from build123d import *

# Parameters (mm, degrees)
F1_DEPTH = 18.288
F2_W     = 17.783007
F2_H     = 7.712702
F3_DEPTH = 8.6106
F4_R     = 5.08


with BuildPart() as f1:
    # F0 (on Front) → F1 (new body)
    with BuildSketch(Plane.XZ):
        Polygon((-13.85931, 24.089288), (-28.41359, 12.499769), (-15.476452, -17.956408), (28.639189, -30.43874), (20.909246, 14.251674), align=None)
    extrude(amount=F1_DEPTH)

    # F2 (on face) → F3 (join)
    with BuildSketch(Plane(origin=(5.283426, 0, 18.672932), x_dir=(0.962224, 0, -0.272257), z_dir=(0.272257, 0, 0.962224))):
        with Locations((-2.849124, -6.417316)):
            Rectangle(F2_W, F2_H)
    extrude(amount=F3_DEPTH)

    # F4
    f4_edges = [f1.edges().sort_by_distance(p)[0] for p in [
        (3.524968, -18.288, 19.170481),
    ]]
    fillet(f4_edges, radius=F4_R)


solid = f1.part
Work out the finished part from the listing and answer in its coordinate system (mm). A direction names the side the tool comes from. Give positions to 0.01 mm unless a question says otherwise; leave off trailing zeros. Loops run counter-clockwise (first coordinate to the right, second up) from the corner with the lowest first, then second, coordinate; pieces in that order, holes last. Notation, with made-up numbers: (-10.75, 53) - (2.25, 53) arc R21 ccw to (2.25, 68) - close; hole circle Ø7 at (-19, 52.5). An arc over 180 degrees is marked (long way). Answer in a Markdown table with one row per item. Add a question column.
Q1. The part is cut by section C-C (z = -24.5). Determine the outline of the cut face in (x, y).
Q2. Determine the mould class of faces 1 (the flat face through (12.253, -6.471, 21.113)), 2 (the flat face through (-22.036, -9.016, -2.515)), 3 (the flat face through (-4.86, -6.47, 25.95)), 4 (the flat face through (4, -10.274, 24)) for opening direction X: released by +X, released by -X, zero draft, split by the parting line, or undercut.
Q3. Each of these flat-tipped pins is pushed along its axis until it touches: P1, Ø6, axis at y = -7.5, z = -14.5, coming from the +X side; P2, Ø1.5, axis at x = -8.5, z = 21, coming from the -Y side; P3, Ø10.5, axis at x = 8, z = 25, coming from the +Y side. Where does it stop, or does it pass through?
Q4. The part is cut by section A-A (y = -9.5). Determine the outline of the cut face in (x, z), and give its area (3 significant figures).
Q5. Consider line 1 along Y through (x, z) = (-12, 21.5); line 2 along X through (y, z) = (-11.25, 0); line 3 along Z through (x, y) = (-11, -9.5). Determine where each line is inside the solid, lowest interval first.
Q6. A tool of negligible diameter and unlimited length cuts with its end or side. For faces 5 (the cylindrical face through (2.263, -16.76, 18.022)), 6 (the flat face through (4, -2.561, 24)), from which of +Z, -Z, +X, -X, +Y, -Y can it reach the whole face along a straight path? Write none if from no direction.
Q7. The part is cut by section B-B (z = -7). Determine the outline of the cut face in (x, y), and give its area (3 significant figures).
Solution:
| question | item | result |
|---|---|---|
| 1 | outline | (7.65, -18.29) - (27.61, -18.29) - (27.61, 0) - (7.65, 0) - close |
| 2 | face 1 | released by +X |
| 2 | face 2 | released by -X |
| 2 | face 3 | undercut |
| 2 | face 4 | zero draft |
| 3 | P1 | stops at x = 26.4 |
| 3 | P2 | stops at y = -17.44 |
| 3 | P3 | stops at y = -2.56 |
| 4 | outline | (-28.41, 12.5) - (-15.48, -17.96) - (28.64, -30.44) - (20.91, 14.25) - (11.1, 17.03) - (13.44, 25.31) - (-3.67, 30.15) - (-6.01, 21.87) - (-13.86, 24.09) - close |
| 4 | area | 2,130 mm² |
| 5 | line 1 | y = -17.24 to 0 |
| 5 | line 2 | x = -23.1 to 23.37 |
| 5 | line 3 | z = -19.22 to 23.28 |
| 6 | face 5 | +Z, +X, -Y |
| 6 | face 6 | +Z, +X, +Y |
| 7 | outline | (-20.13, -18.29) - (24.59, -18.29) - (24.59, 0) - (-20.13, 0) - close |
| 7 | area | 818 mm² |
